Here's how the part is built. I have some questions about the finished solid (model axes, mm). Face numbers are marked on the shaded views. A direction names the side the tool comes from. Round coordinates to 2 decimals unless told otherwise and drop trailing zeros. Write each loop counter-clockwise with the first axis right and the second up, starting at its lowest first coordinate (ties: lowest second). Pieces come first, ordered by that corner, then holes. Notation, with made-up numbers: (49.25, -32) -> (73.25, -32) arc R29 cw to (73.25, -10) -> close; hole circle Ø7 at (62.5, -9.5). An arc over 180 degrees is marked (long way). Answer in a Markdown table with one row per item.
from build123d import *

# Parameters (mm, degrees)
F1_DEPTH = 15
F2_DEPTH = 15
F3_R     = 9.4573598756
F3_R_2   = 7.62
F4_DEPTH = 20
F5_R     = 9.6111895613
F5_R_2   = 7.62
F6_DEPTH = 20


with BuildPart() as f1:
    # F0 (on Top) → F1 (new body)
    with BuildSketch(Plane.XY):
        Polygon((-83.9506240486, -25.2640620153), (-57.5444474816, -26.0300338268), (-7.5654697983, -27.4797888861), (-6.9855677746, -7.4881978128), (-57.5444474816, -6.0216213632), (-4.2142863446, 22.7399175335), (-13.707871997, 40.3430942769), (-83.9506240486, 2.4604102147), align=None)
    extrude(amount=F1_DEPTH)

    # F2 (add): a face of the model
    f2_faces = [f1.faces().sort_by_distance(p)[0] for p in [
        (-48.3323554586, 20.4804051436, 0),
    ]]
    extrude(f2_faces, amount=F2_DEPTH)

    # F3 (on face) → F4 (join)
    with BuildSketch(Plane(origin=(6.235860558, 3.3630677682, 0), x_dir=(-0.4746792826, 0.8801588372, 0), z_dir=(0.8801588372, 0.4746792826, 0))):
        with Locations((32.0151737925, 0)):
            Circle(F3_R)
        with Locations((32.0151737925, 0)):
            Circle(F3_R_2, mode=Mode.SUBTRACT)
    extrude(amount=F4_DEPTH)

    # F5 (on face) → F6 (join)
    with BuildSketch(Plane(origin=(-6.7626651312, 0.1961666373, 0), x_dir=(0.0289951012, 0.9995795537, 0), z_dir=(0.9995795537, -0.0289951012, 0))):
        with Locations((-17.5103756727, -0.2658314989)):
            Circle(F5_R)
        with Locations((-17.5103756727, -0.2658314989)):
            Circle(F5_R_2, mode=Mode.SUBTRACT)
    extrude(amount=F6_DEPTH)


solid = f1.part
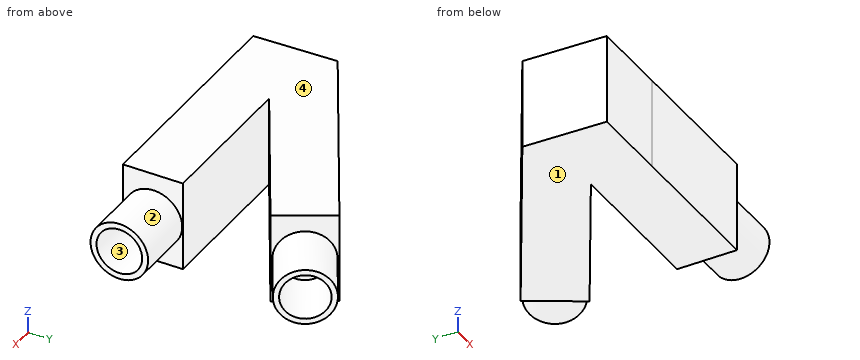
1) I want a section at A-A, the plane x = -55. List the corners of the cut face in (y, z) for me.
Response:
| item | result |
|---|---|
| outline | (-26.1, -15) -> (-6.1, -15) -> (-6.1, 15) -> (-26.1, 15) -> close; (-4.65, -15) -> (18.07, -15) -> (18.07, 15) -> (-4.65, 15) -> close |
2) Which directions (+Z, -Z, +X, -X, +Y, -Y) give clear straight access to the entire face, cutting with the end or side of a thin tool? Please do the marked faces 1 and 2.
Response:
| item | result |
|---|---|
| face 1 | -Z, +X, -X, +Y, -Y |
| face 2 | none |
3) I need wall thicknesses on line 1 (Z direction, x = -7, y = 36.5); line 2 (X direction, y = 32.5, z = 0.5); line 3 (X direction, y = 35, z = -3.75). Which ranges of each line are inside material? Lowest first, please. Write a range as [from, to].
Response:
| item | result |
|---|---|
| line 1 | z = [-8.81, -6.8], [6.8, 8.81] |
| line 2 | x = [-28.25, -9.48], [8.83, 12.71] |
| line 3 | x = [-23.62, -10.83], [11.43, 11.9] |
4) We'd pull the mould along Y, two halves only. Please class the marked faces 3 and 4: +Y half, -Y half, draft (parallel to the pull), parting line (faces both ways), or undercut.
Response:
| item | result |
|---|---|
| face 3 | undercut |
| face 4 | draft |
5) For pin 1 (4 mm diameter, centred on x = -55.5, z = -11.5, fed in from -Y); pin 2 (10 mm diameter, centred on x = -64, z = 7, fed in from -Y); pin 3 (3 mm diameter, centred on x = -40.5, z = 7.5, fed in from -Y); pin 4 (8 mm diameter, centred on x = -43.5, y = 33, fed in from -Z), each with a flat end and sliding along its axis, tell me the tip position at first contact or that it passes through.
Response:
| item | result |
|---|---|
| pin 1 | stops at y = -26.15 |
| pin 2 | stops at y = -25.99 |
| pin 3 | stops at y = -26.57 |
| pin 4 | passes through |
6) I want a section at C-C, the plane x = -9. Count the separate pieces of the cut face and the enclosed holes in it, and give its area (4 significant figures).
Response:
| item | result |
|---|---|
| separate pieces | 2 |
| enclosed holes | 1 |
| area | 1,000 mm^2 |
7) I want a section at D-D, the plane y = 9. List the corners of the cut face in (x, z) for me, and give its area (3 significant figures).
Response:
| item | result |
|---|---|
| outline | (-71.82, -15) -> (-29.69, -15) -> (-29.69, 15) -> (-71.82, 15) -> close |
| area | 1,260 mm^2 |
8) I want a section at B-B, the plane z = 11. List the corners of the cut face in (x, y) for me.
Response:
| item | result |
|---|---|
| outline | (-83.95, -25.26) -> (-7.57, -27.48) -> (-6.99, -7.49) -> (-57.54, -6.02) -> (-4.21, 22.74) -> (-13.71, 40.34) -> (-83.95, 2.46) -> close |
